```python
from build123d import *

# Parameters (mm, degrees)
Y_KSEKLIK_EKSTR_ZYON1_DEPTH = 3.24
IZIM2_W                     = 1.429951724
IZIM2_H                     = 0.588312172
KES_EKSTR_ZYON1_DEPTH       = 1.04186858
KES_EKSTR_ZYON2_DEPTH       = 0.5
Y_KSEKLIK_EKSTR_ZYON2_DEPTH = 0.3


with BuildPart() as part:
    # Çizim1 → Yükseklik-Ekstrüzyon1 (new, symmetric)
    with BuildSketch(Plane.XY):
        with BuildLine():
            Line((-0.3, 0.35), (-0.3, 13.55))
            ThreePointArc((-0.3, 13.55), (0.546641464, 14.640795493), (1.813383319, 14.091248725))
            Line((1.813383319, 14.091248725), (3.870705293, 10.338139841))
            ThreePointArc((3.870705293, 10.338139841), (3.952443157, 10.131139603), (3.9802691, 9.910332234))
            Line((3.9802691, 9.910332234), (3.9802691, 7.110332234))
            Line((3.9802691, 7.110332234), (3.6802691, 7.110332234))
            Line((3.6802691, 7.110332234), (3.6802691, 9.910332234))
            ThreePointArc((3.6802691, 9.910332234), (3.661822688, 10.056710153), (3.607636913, 10.19393503))
            Line((3.607636913, 10.19393503), (1.550314939, 13.947043914))
            ThreePointArc((1.550314939, 13.947043914), (0.621070914, 14.350175024), (0, 13.55))
            Line((0, 13.55), (0, 0.35))
            ThreePointArc((0, 0.35), (-0.102512627, 0.102512627), (-0.35, 0))
            Line((-0.35, 0), (-7.3, 0))
            Line((-7.3, 0), (-7.3, 0.3))
            Line((-7.3, 0.3), (-0.35, 0.3))
            ThreePointArc((-0.35, 0.3), (-0.314644661, 0.314644661), (-0.3, 0.35))
        make_face()
    extrude(amount=Y_KSEKLIK_EKSTR_ZYON1_DEPTH, both=True)

    # Çizim2 → Kes-Ekstrüzyon1 (cut)
    with BuildSketch(Plane(origin=(0, 0, 0), x_dir=(1, 0, 0), z_dir=(0, 1, 0))):
        Polygon((0, -4), (0, -1.778), (-2.671699332, -1.778), (-2.671699332, -3.175), (-7.3, -3.175), (-7.3, 3.175), (-2.671699332, 3.175), (-2.671699332, 1.778), (0, 1.778), (0, 4), (-8, 4), (-8, -4), align=None)
        with Locations((-5.68100521, 0)):
            Rectangle(IZIM2_W, IZIM2_H)
    extrude(amount=KES_EKSTR_ZYON1_DEPTH, mode=Mode.SUBTRACT)

    # Çizim4 → Kes-Ekstrüzyon2 (cut)
    with BuildSketch(Plane(origin=(0, 0, 0), x_dir=(0, 0, -1), z_dir=(1, 0, 0))):
        with BuildLine():
            Line((-0.55, -0.15), (0.55, -0.15))
            Line((0.55, -0.15), (0.55, 0.33))
            ThreePointArc((0.55, 0.33), (0.544142136, 0.344142136), (0.53, 0.35))
            Line((0.53, 0.35), (-0.53, 0.35))
            ThreePointArc((-0.53, 0.35), (-0.544142136, 0.344142136), (-0.55, 0.33))
            Line((-0.55, 0.33), (-0.55, -0.15))
        make_face()
    extrude(amount=-KES_EKSTR_ZYON2_DEPTH, mode=Mode.SUBTRACT)

    # Çizim5 → Yükseklik-Ekstrüzyon2 (add)
    with BuildSketch(Plane(origin=(0, 0, 0), x_dir=(0, 0, -1), z_dir=(1, 0, 0))):
        with BuildLine():
            Line((-0.51, -0.22), (0.51, -0.22))
            Line((0.51, -0.22), (0.51, 0.33))
            ThreePointArc((0.51, 0.33), (0.515857864, 0.344142136), (0.53, 0.35))
            Line((0.53, 0.35), (-0.53, 0.35))
            ThreePointArc((-0.53, 0.35), (-0.515857864, 0.344142136), (-0.51, 0.33))
            Line((-0.51, 0.33), (-0.51, -0.22))
        make_face()
    extrude(amount=-Y_KSEKLIK_EKSTR_ZYON2_DEPTH)


solid = part.part
```
Can you work these out from the model? Positions are in its coordinate system, mm. A direction names the side the tool comes from. Give positions to 0.01 mm unless a question says otherwise; leave off trailing zeros. Order: outer loops, then holes, each group sorted by start corner. A loop starts at its lowest first (then second) coordinate and runs counter-clockwise, first axis right, second up. Notation, with made-up numbers: (-25.75, -30.5) - (-5.75, -30.5) arc R33 cw to (-5.75, -0.5) - close; hole circle Ø6 at (26, 6.25). An arc over 180 degrees is marked (long way). Use a Markdown table: item, result. Add a question column.
Q1. If we section it at A-A on z = 0: Write out the boundary of the cut face in (x, y).
Q2. Please list where these lines run through material, in increasing order: line 1 along X through (y, z) = (7.5, -2.25); line 2 along Y through (x, z) = (-6.25, -1.5); line 3 along X through (y, z) = (6, 1).
Q3. If we section it at D-D on x = -5.5: Write out the boundary of the cut face in (y, z) (3 decimals), plus the area to 3 significant figures.
Q4. If we section it at B-B on z = 2.75: Write out the boundary of the cut face in (x, y), plus the area to 3 significant figures.
Q5. I'm going to push flat-ended pins straight in: pin 1 (3 mm diameter, centred on x = -4.5, z = 1.5, fed in from +Y); pin 2 (3 mm diameter, centred on y = 7, z = 1.5, fed in from -X); pin 3 (3 mm diameter, centred on x = -2.5, z = 0.5, fed in from -Y). Where does each tip first touch, or does it pass through?
Q6. If we section it at C-C on y = 8: Write out the boundary of the cut face in (x, z).
Q7. On a 3-axis mill with a long thin cutter (end or side, diameter ignored), from which of +Z, -Z, +X, -X, +Y, -Y can I reach the whole of each face in a straight line? I mean faces 1 (the flat face through (3.98, 9, 0)), 2 (the flat face through (-4, 0.3, 0)), 3 (the flat face through (2.593, 12.044, 0.045)). Say none if no direction works.
Answers follow:
| question | item | result |
|---|---|---|
| 1 | outline | (-7.3, 0) - (-6.4, 0) - (-6.4, 0.3) - (-7.3, 0.3) - close; (-4.97, 0) - (-0.5, 0) - (-0.5, 0.3) - (-4.97, 0.3) - close; (-0.3, -0.22) - (0, -0.22) - (0, 13.55) arc R0.83 cw to (1.55, 13.95) - (3.61, 10.19) arc R0.59 cw to (3.68, 9.91) - (3.68, 7.11) - (3.98, 7.11) - (3.98, 9.91) arc R0.89 ccw to (3.87, 10.34) - (1.81, 14.09) arc R1.13 ccw to (-0.3, 13.55) - close |
| 2 | line 1 | x = -0.3 to 0, 3.68 to 3.98 |
| 2 | line 2 | y = 0 to 0.3 |
| 2 | line 3 | x = -0.3 to 0 |
| 3 | outline | (0, -3.175) - (0.3, -3.175) - (0.3, -0.294) - (0, -0.294) - close; (0, 0.294) - (0.3, 0.294) - (0.3, 3.175) - (0, 3.175) - close |
| 3 | area | 1.73 mm^2 |
| 4 | outline | (-7.3, 0) - (-2.67, 0) - (-2.67, 0.3) - (-7.3, 0.3) - close; (-0.3, 1.04) - (0, 1.04) - (0, 13.55) arc R0.83 cw to (1.55, 13.95) - (3.61, 10.19) arc R0.59 cw to (3.68, 9.91) - (3.68, 7.11) - (3.98, 7.11) - (3.98, 9.91) arc R0.89 ccw to (3.87, 10.34) - (1.81, 14.09) arc R1.13 ccw to (-0.3, 13.55) - close |
| 4 | area | 8.15 mm^2 |
| 5 | pin 1 | stops at y = 0.3 |
| 5 | pin 2 | stops at x = -0.3 |
| 5 | pin 3 | stops at y = 0 |
| 6 | outline | (-0.3, -3.24) - (0, -3.24) - (0, 3.24) - (-0.3, 3.24) - close; (3.68, -3.24) - (3.98, -3.24) - (3.98, 3.24) - (3.68, 3.24) - close |
| 7 | face 1 | +Z, -Z, +X, +Y, -Y |
| 7 | face 2 | +Z, -Z, -X, +Y |
| 7 | face 3 | +Z, -Z, -Y |
